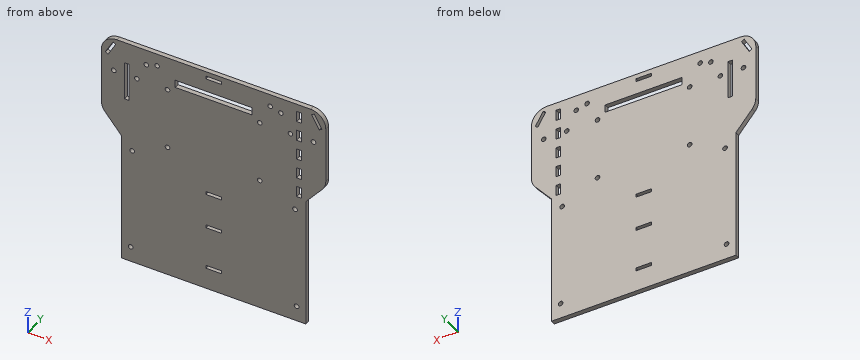
```python
from build123d import *

# Parameters (mm, degrees)
BOSS_EXTRUDE1_DEPTH = 3
SKETCH2_R           = 1.525
CUT_EXTRUDE1_DEPTH  = 105.70434566
SKETCH3_W           = 10
SKETCH3_H           = 2.05
CUT_EXTRUDE2_DEPTH  = 105.70434566
SKETCH4_R           = 1.5
CUT_EXTRUDE3_DEPTH  = 3
SKETCH5_R           = 1.5
SKETCH5_R_2         = 1.525
SKETCH5_W           = 50
SKETCH5_H           = 5
CUT_EXTRUDE4_DEPTH  = 3
SKETCH6_W           = 3.05
SKETCH6_H           = 7
CUT_EXTRUDE5_DEPTH  = 10
SKETCH7_W           = 10
SKETCH7_H           = 2
SKETCH7_W_2         = 3.05
SKETCH7_H_2         = 25
CUT_EXTRUDE6_DEPTH  = 10
FILLET3_R           = 10
CUT_EXTRUDE7_DEPTH  = 10
SKETCH9_R           = 1.5
CUT_EXTRUDE8_DEPTH  = 3


with BuildPart() as part:
    # Sketch1 → Boss-Extrude1 (new body)
    with BuildSketch(Plane(origin=(0, 0, 0), x_dir=(1, 0, 0), z_dir=(0, 1, 0))):
        Polygon((-73, -25), (-60, -9.801315846), (-60, 75), (60, 75), (60, -9.801315846), (73, -25), (73, -75), (60, -75), (-60, -75), (-73, -75), align=None)
    extrude(amount=BOSS_EXTRUDE1_DEPTH)

    # Sketch2 → Cut-Extrude1 (cut, through all)
    with BuildSketch(Plane(origin=(0, 3, 0), x_dir=(1, 0, 0), z_dir=(0, 1, 0))):
        with Locations(Location((-53, -1.81, 0), (0, 0, 270))):
            Circle(SKETCH2_R)
        with Locations(Location((-54, 65, 0), (0, 0, 270))):
            Circle(SKETCH2_R)
        with Locations(Location((53, -1.81, 0), (0, 0, 90))):
            Circle(SKETCH2_R)
        with Locations(Location((54, 65, 0), (0, 0, 90))):
            Circle(SKETCH2_R)
    extrude(amount=-CUT_EXTRUDE1_DEPTH, mode=Mode.SUBTRACT)

    # Sketch3 → Cut-Extrude2 (cut, through all)
    with BuildSketch(Plane(origin=(0, 3, 0), x_dir=(1, 0, 0), z_dir=(0, 1, 0))):
        with Locations((0, 32.065)):
            Rectangle(SKETCH3_W, SKETCH3_H)
        with Locations((0, 9.015)):
            Rectangle(SKETCH3_W, SKETCH3_H)
        with Locations((0, 60.115)):
            Rectangle(SKETCH3_W, SKETCH3_H)
    extrude(amount=-CUT_EXTRUDE2_DEPTH, mode=Mode.SUBTRACT)

    # Sketch4 → Cut-Extrude3 (cut)
    with BuildSketch(Plane(origin=(0, 3, 0), x_dir=(1, 0, 0), z_dir=(0, 1, 0))):
        with Locations(Location((-50, -53, 0), (0, 0, 270))):
            Circle(SKETCH4_R)
        with Locations(Location((-43.815341562, -65, 0), (0, 0, 270))):
            Circle(SKETCH4_R)
        with Locations(Location((43.815341562, -65, 0), (0, 0, 90))):
            Circle(SKETCH4_R)
        with Locations(Location((50, -53, 0), (0, 0, 90))):
            Circle(SKETCH4_R)
    extrude(amount=-CUT_EXTRUDE3_DEPTH, mode=Mode.SUBTRACT)

    # Sketch5 → Cut-Extrude4 (cut)
    with BuildSketch(Plane(origin=(0, 3, 0), x_dir=(1, 0, 0), z_dir=(0, 1, 0))):
        with Locations(Location((-36.8, -67, 0), (0, 0, 270))):
            Circle(SKETCH5_R)
        with Locations(Location((36.8, -67, 0), (0, 0, 90))):
            Circle(SKETCH5_R)
        with Locations(Location((-65, -53, 0), (0, 0, 270))):
            Circle(SKETCH5_R_2)
        with Locations(Location((65, -53, 0), (0, 0, 90))):
            Circle(SKETCH5_R_2)
        with Locations((0, -59)):
            Rectangle(SKETCH5_W, SKETCH5_H)
    extrude(amount=-CUT_EXTRUDE4_DEPTH, mode=Mode.SUBTRACT)

    # Sketch6 → Cut-Extrude5 (cut)
    with BuildSketch(Plane(origin=(0, 3, 0), x_dir=(1, 0, 0), z_dir=(0, 1, 0))):
        with Locations((55.525, -53.5)):
            Rectangle(SKETCH6_W, SKETCH6_H)
        with Locations((55.525, -66.5)):
            Rectangle(SKETCH6_W, SKETCH6_H)
        with Locations((55.525, -40.5)):
            Rectangle(SKETCH6_W, SKETCH6_H)
        with Locations((55.525, -27.5)):
            Rectangle(SKETCH6_W, SKETCH6_H)
        with Locations((55.525, -14.5)):
            Rectangle(SKETCH6_W, SKETCH6_H)
    extrude(amount=-CUT_EXTRUDE5_DEPTH, mode=Mode.SUBTRACT)

    # Sketch7 → Cut-Extrude6 (cut)
    with BuildSketch(Plane(origin=(0, 3, 0), x_dir=(1, 0, 0), z_dir=(0, 1, 0))):
        with Locations((0, -71)):
            Rectangle(SKETCH7_W, SKETCH7_H)
        with Locations((-56.475, -48.5)):
            Rectangle(SKETCH7_W_2, SKETCH7_H_2)
    extrude(amount=-CUT_EXTRUDE6_DEPTH, mode=Mode.SUBTRACT)

    # Fillet3
    fillet3_edges = [part.edges().sort_by_distance(p)[0] for p in [
        (73, 1.5, 25),
        (73, 1.5, 75),
        (-73, 1.5, 75),
        (-73, 1.5, 25),
    ]]
    fillet(fillet3_edges, radius=FILLET3_R)

    # Sketch8 → Cut-Extrude7 (cut)
    with BuildSketch(Plane(origin=(0, 3, 0), x_dir=(1, 0, 0), z_dir=(0, 1, 0))):
        Polygon((70.5, -63.839745962), (65.5, -72.5), (63.724647922, -71.475), (68.724647922, -62.814745962), align=None)
        Polygon((-68.724647922, -62.814745962), (-70.5, -63.839745962), (-65.5, -72.5), (-63.724647922, -71.475), align=None)
    extrude(amount=-CUT_EXTRUDE7_DEPTH, mode=Mode.SUBTRACT)

    # Sketch9 → Cut-Extrude8 (cut)
    with BuildSketch(Plane(origin=(0, 3, 0), x_dir=(1, 0, 0), z_dir=(0, 1, 0))):
        with Locations(Location((-30, -13, 0), (0, 0, 270))):
            Circle(SKETCH9_R)
        with Locations(Location((30, -13, 0), (0, 0, 90))):
            Circle(SKETCH9_R)
        with Locations(Location((30, -53, 0), (0, 0, 270))):
            Circle(SKETCH9_R)
        with Locations(Location((-30, -53, 0), (0, 0, 90))):
            Circle(SKETCH9_R)
    extrude(amount=-CUT_EXTRUDE8_DEPTH, mode=Mode.SUBTRACT)


solid = part.part
```
Read the model definition and answer for the solid it produces. Units are mm, in the model's axes. Give positions to 0.01 mm unless a question says otherwise; leave off trailing zeros. Write each loop counter-clockwise with the first axis right and the second up, starting at its lowest first coordinate (ties: lowest second). Pieces come first, ordered by that corner, then holes. Notation, with made-up numbers: M -7,-2.75 L 46,-2.75 A27 cw 46,35.25 Z; hole C 27.5,30.25 d2. An arc over 180 degrees is marked long. Put each result on its own line as item: value. Start each with the question number.
1. The part is cut by section D-D, the plane y = 1.3. Give the number of separate pieces and of enclosed holes in the cut face, and give its area (3 significant figures).
2. The part is cut by section B-B, the plane x = 8. Give the vertices of the cut face in (y, z), and give its area (3 significant figures).
3. The part is cut by section C-C, the plane z = -47. Give the vertices of the cut face in (x, y), and give its area (3 significant figures).
4. Consider line 1 along X through (y, z) = (0.9, 1.81) (3 decimals); line 2 along Z through (x, y) = (-24, 2.25); line 3 along X through (y, z) = (1.4, 67). Determine where each line is inside the solid, lowest interval first.
5. Each of these flat-tipped pins is pushed along its axis until it touches: pin 1 Ø2 at (x, z) = (-34, 10) entering from -Y; pin 2 Ø1.6 at (y, z) = (2, -32) entering from -X; pin 3 Ø1 at (y, z) = (0.5, -28.5) entering from +X; pin 4 Ø0.9 at (y, z) = (1, 14.5) entering from -X. Where does it stop, or does it pass through?
6. The part is cut by section A-A, the plane z = 46.5. Give the vertices of the cut face in (x, y), and give its area (3 significant figures).
Final values:
1. separate pieces: 1
1. enclosed holes: 29
1. area: 18,800 mm²
2. outline: M 0,-75 L 3,-75 L 3,56.5 L 0,56.5 Z; M 0,61.5 L 3,61.5 L 3,75 L 0,75 Z
2. area: 435 mm²
3. outline: M -60,0 L 60,0 L 60,3 L -60,3 Z
3. area: 360 mm²
4. line 1: x = -60 to -54.525, -51.475 to 51.475, 54.525 to 60
4. line 2: z = -75 to 56.5, 61.5 to 75
4. line 3: x = -72.8 to -68.68, -66.31 to -38.3, -35.3 to 35.3, 38.3 to 54, 57.05 to 66.31, 68.68 to 72.8
5. pin 1: stops at y = 0
5. pin 2: stops at x = -60
5. pin 3: stops at x = 60
5. pin 4: stops at x = -64.4
6. outline: M -73,0 L -58,0 L -58,3 L -73,3 Z; M -54.95,0 L 73,0 L 73,3 L -54.95,3 Z
6. area: 429 mm²
